Build history of the part. All positions in model axes, mm. Face numbers are marked on the shaded views. A direction names the side the tool comes from. Round coordinates to 2 decimals unless told otherwise and drop trailing zeros. Loops run counter-clockwise (first coordinate to the right, second up) from the corner with the lowest first, then second, coordinate; pieces in that order, holes last. Notation, with made-up numbers: (77, 82.5) - (103, 82.5) arc R30 cw to (103, 107.5) - close; hole circle Ø4 at (85, -37). An arc over 180 degrees is marked (long way). Put each result on its own line as item: value. Start each with the question number.
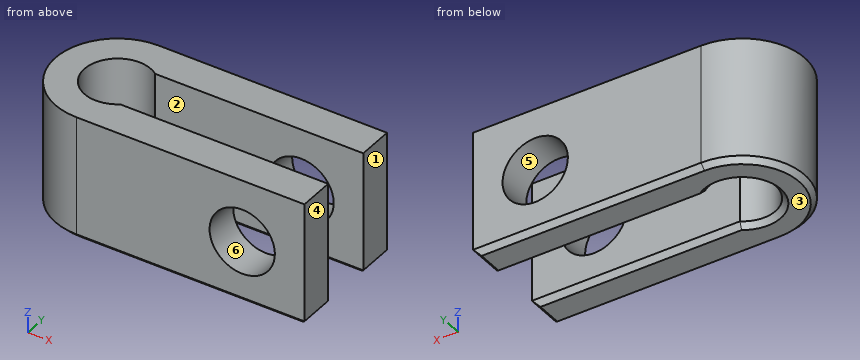
from build123d import *

# Parameters (mm, degrees)
BOSS_EXTRUDE1_DEPTH     = 12
CUT_EXTRUDE1_DEPTH      = 26.768197453
CUT_EXTRUDE1_DEPTH_BACK = 26.768197453
SKETCH2_R               = 3.15
CHAMFER1_SIZE           = 0.5


with BuildPart() as part:
    # Sketch1 → Boss-Extrude1 (new body)
    with BuildSketch(Plane.XY):
        with BuildLine():
            Line((0, 6), (22, 6))
            Line((22, 6), (22, 2.552710574))
            Line((22, 2.552710574), (1.929680991, 2.552710574))
            ThreePointArc((1.929680991, 2.552710574), (-3.2, 0), (1.929680991, -2.552710574))
            Line((1.929680991, -2.552710574), (22, -2.552710574))
            Line((22, -2.552710574), (22, -6))
            Line((22, -6), (0, -6))
            ThreePointArc((0, -6), (-6, 0), (0, 6))
        make_face()
    extrude(amount=BOSS_EXTRUDE1_DEPTH)

    # Sketch2 → Cut-Extrude1 (cut, two sides: drawn at the far end of the back side and taken through both)
    with BuildSketch(Plane(origin=(0, 0, 0), x_dir=(1, 0, 0), z_dir=(0, 1, 0)).offset(-CUT_EXTRUDE1_DEPTH_BACK)):
        with Locations(Location((16, -6, 0), (0, 0, 270))):
            Circle(SKETCH2_R)
    extrude(amount=CUT_EXTRUDE1_DEPTH + CUT_EXTRUDE1_DEPTH_BACK, mode=Mode.SUBTRACT)

    # Chamfer1
    chamfer1_edges = [part.edges().sort_by_distance(p)[0] for p in [
        (11.964840496, 2.552710574, 0),
        (-3.2, 0, 0),
        (11.964840496, -2.552710574, 0),
        (22, -4.276355287, 0),
        (11, -6, 0),
        (-6, 0, 0),
        (11, 6, 0),
        (22, 4.276355287, 0),
    ]]
    chamfer(chamfer1_edges, length=CHAMFER1_SIZE)


solid = part.part
Item 1: Which spindle directions (+Z, -Z, +X, -X, +Y, -Y) get a long thin tool onto all of the face, cutting with end or side? Do the marked faces 1 and 2. Say none if no direction does.
Item 2: Drill centre lines: probe 1 along Y at (x, z) = (16.75, 2.5); probe 2 along Z at (x, y) = (16, 3.75); probe 3 along Y at (x, z) = (0, 11.25). Where is each one in solid material? Low to high. Write a range as [from, to].
Item 3: Slice it at C-C (z = 6). Give the cut face in (x, y).
Item 4: Drop flat-ended pins along their axis: pin 1 Ø3 at (x, y) = (5, -1.5) entering from -Z; pin 2 Ø3 at (y, z) = (4, 3.5) entering from -X. Give the stop position or say it passes through.
Item 5: Slice it at B-B (x = 16). Give the cut face in (y, z).
Item 6: Slice it at A-A (x = 12.5). Give the cut face in (y, z).
Item 7: Slice it at D-D (z = 10.75). Give the cut face in (x, y), plus the area to 3 significant figures.
Item 8: Two-plate mould, pull along Z, no slides. Class the marked faces 3, 4, 5 and 6: pulls with the +Z half, pulls with the -Z half, needs draft (parallel to the pull), parting line crosses it, or undercut.
Computed values:
1. face 1: +Z, -Z, +X, +Y, -Y
1. face 2: +Z, -Z, +X
2. probe 1: y = [-6, -2.55], [2.55, 6]
2. probe 2: z = [0, 2.85], [9.15, 12]
2. probe 3: y = [-6, -3.2], [3.2, 6]
3. outline: (0, -6) - (12.85, -6) - (12.85, -2.55) - (1.93, -2.55) arc R3.2 cw (long way) to (1.93, 2.55) - (12.85, 2.55) - (12.85, 6) - (0, 6) arc R6 ccw to start; (19.15, -6) - (22, -6) - (22, -2.55) - (19.15, -2.55) - close; (19.15, 2.55) - (22, 2.55) - (22, 6) - (19.15, 6) - close
4. pin 1: stops at z = 0.05
4. pin 2: stops at x = -5.45
5. outline: (-6, 0.5) - (-5.5, 0) - (-3.05, 0) - (-2.55, 0.5) - (-2.55, 2.85) - (-6, 2.85) - close; (-6, 9.15) - (-2.55, 9.15) - (-2.55, 12) - (-6, 12) - close; (2.55, 0.5) - (3.05, 0) - (5.5, 0) - (6, 0.5) - (6, 2.85) - (2.55, 2.85) - close; (2.55, 9.15) - (6, 9.15) - (6, 12) - (2.55, 12) - close
6. outline: (-6, 0.5) - (-5.5, 0) - (-3.05, 0) - (-2.55, 0.5) - (-2.55, 12) - (-6, 12) - close; (2.55, 0.5) - (3.05, 0) - (5.5, 0) - (6, 0.5) - (6, 12) - (2.55, 12) - close
7. outline: (0, -6) - (22, -6) - (22, -2.55) - (1.93, -2.55) arc R3.2 cw (long way) to (1.93, 2.55) - (22, 2.55) - (22, 6) - (0, 6) arc R6 ccw to start
7. area: 190 mm^2
8. face 3: pulls with the -Z half
8. face 4: needs draft
8. face 5: undercut
8. face 6: undercut
